The listing builds one solid part. Answer for the finished solid, in the listing's coordinates (mm). A direction names the side the tool comes from. Give positions to 0.01 mm unless a question says otherwise; leave off trailing zeros. Write each loop counter-clockwise with the first axis right and the second up, starting at its lowest first coordinate (ties: lowest second). Pieces come first, ordered by that corner, then holes. Notation, with made-up numbers: M 34.5,52 L 48.5,52 A21 ccw 48.5,63 Z; hole C 19.5,36 d10. An arc over 180 degrees is marked long. Return JSON: item names as keys, results as strings.
from build123d import *

# Parameters (mm, degrees)
SKETCH1_W             = 35.56
SKETCH1_H             = 35.56
BOSS_EXTRUDE1_DEPTH   = 6.35
CUT_EXTRUDE1_DEPTH    = 2.921
LPATTERN11_COUNT      = 2
LPATTERN11_PITCH      = 35.56
LPATTERN11_COUNT_DIR2 = 2
LPATTERN11_PITCH_DIR2 = 35.56
LPATTERN15_COUNT      = 2
LPATTERN15_PITCH      = 35.56
LPATTERN16_COUNT      = 2
LPATTERN16_PITCH      = 35.56
SKETCH20_W            = 3.175
SKETCH20_H            = 12.7
BOSS_EXTRUDE2_DEPTH   = 6.35
CUT_EXTRUDE2_DEPTH    = 76.700949135
SKETCH22_W            = 12.7
SKETCH22_H            = 3.175
BOSS_EXTRUDE3_DEPTH   = 6.35
CUT_EXTRUDE3_DEPTH    = 78.97065682
CUT_EXTRUDE4_DEPTH    = 78.97065682
CUT_EXTRUDE5_DEPTH    = 78.97065682


with BuildPart() as part:
    # Sketch1 → Boss-Extrude1 (new body)
    with BuildSketch(Plane(origin=(0, 0, 0), x_dir=(1, 0, 0), z_dir=(0, 1, 0))):
        Rectangle(SKETCH1_W, SKETCH1_H)
    boss_extrude1 = extrude(amount=BOSS_EXTRUDE1_DEPTH)

    # Sketch2 → Cut-Extrude1 (cut)
    with BuildSketch(Plane(origin=(0, 6.35, 0), x_dir=(1, 0, 0), z_dir=(0, 1, 0))):
        Polygon((0, 6.599113577), (-5.715, 3.299556788), (-5.715, -3.299556788), (0, -6.599113577), (5.715, -3.299556788), (5.715, 3.299556788), align=None)
    cut_extrude1 = extrude(amount=-CUT_EXTRUDE1_DEPTH, mode=Mode.SUBTRACT)

    # Sketch3 → 1/4 Clearance Hole1 (revolve, cut)
    with BuildSketch(Plane(origin=(0, 3.429, 0), x_dir=(0, 0, 1), z_dir=(1, 0, 0))):
        Polygon((0, 0), (0, 11.035817477), (3.57124, 8.89), (3.57124, 0), align=None)
    f_1_4_clearance_hole1 = revolve(axis=Axis((0, 9.779, 0), (0, -1, 0)), mode=Mode.SUBTRACT)

    # LPattern11: Boss-Extrude1, Cut-Extrude1, 1_4 Clearance Hole1 2 × 2
    with Locations(*[(-j * LPATTERN11_PITCH_DIR2, 0, i * LPATTERN11_PITCH) for i in range(LPATTERN11_COUNT) for j in range(LPATTERN11_COUNT_DIR2) if (i, j) != (0, 0)]):
        add(boss_extrude1)
        add(cut_extrude1, mode=Mode.SUBTRACT)
        add(f_1_4_clearance_hole1, mode=Mode.SUBTRACT)

    # Sketch15 → CBORE for #4 Socket Head Cap Screw5 (revolve, cut)
    with BuildSketch(Plane(origin=(0, 0, -11.557), x_dir=(0, 0, -1), z_dir=(1, 0, 0))):
        Polygon((0, 0), (0, 9.775187864), (1.4732, 8.89), (1.4732, 3.81), (2.794, 3.81), (2.794, 0), align=None)
    cbore_for_4_socket_head_cap_screw5 = revolve(axis=Axis((0, -6.35, -11.557), (0, 1, 0)), mode=Mode.SUBTRACT)

    # LPattern15: CBORE for #4 Socket Head Cap Screw5 ×2
    with Locations(*[(-i * LPATTERN15_PITCH, 0, 0) for i in range(1, LPATTERN15_COUNT)]):
        add(cbore_for_4_socket_head_cap_screw5, mode=Mode.SUBTRACT)

    # Sketch17 → CBORE for #4 Socket Head Cap Screw6 (revolve, cut)
    with BuildSketch(Plane(origin=(0, 0, 17.78), x_dir=(0, 0, -1), z_dir=(1, 0, 0))):
        Polygon((0, 0), (0, 9.775187864), (1.4732, 8.89), (1.4732, 3.81), (2.794, 3.81), (2.794, 0), align=None)
    cbore_for_4_socket_head_cap_screw6 = revolve(axis=Axis((0, -6.35, 17.78), (0, 1, 0)), mode=Mode.SUBTRACT)

    # LPattern16: CBORE for #4 Socket Head Cap Screw6 ×2
    with Locations(*[(-i * LPATTERN16_PITCH, 0, 0) for i in range(1, LPATTERN16_COUNT)]):
        add(cbore_for_4_socket_head_cap_screw6, mode=Mode.SUBTRACT)

    # Mirror1: CBORE for #4 Socket Head Cap Screw5 across plane
    add(cbore_for_4_socket_head_cap_screw5.mirror(Plane.XY.offset(17.78)), mode=Mode.SUBTRACT)

    # Mirror1 copy 1 sketch → Mirror1 copy 1 (revolve, cut)
    with BuildSketch(Plane(origin=(-35.56, 0, 47.117), x_dir=(0, 0, 1), z_dir=(1, 0, 0))):
        Polygon((0, 0), (0, -9.775187864), (1.4732, -8.89), (1.4732, -3.81), (2.794, -3.81), (2.794, 0), align=None)
    revolve(axis=Axis((-35.56, -6.35, 47.117), (0, -1, 0)), mode=Mode.SUBTRACT)

    # Sketch20 → Boss-Extrude2 (add)
    with BuildSketch(Plane(origin=(0, 0, 0), x_dir=(1, 0, 0), z_dir=(0, 1, 0))):
        with Locations((19.3675, 0)):
            Rectangle(SKETCH20_W, SKETCH20_H)
        with Locations((19.3675, -35.56)):
            Rectangle(SKETCH20_W, SKETCH20_H)
    extrude(amount=BOSS_EXTRUDE2_DEPTH)

    # Sketch21 → Cut-Extrude2 (cut, through all)
    with BuildSketch(Plane(origin=(0, 6.35, 0), x_dir=(1, 0, 0), z_dir=(0, 1, 0))):
        Polygon((20.955, -6.35), (17.78, -6.35), (17.78, -3.302), align=None)
        Polygon((20.955, 6.35), (17.78, 6.35), (17.78, 3.302), align=None)
        Polygon((20.955, -29.21), (17.78, -29.21), (17.78, -32.258), align=None)
        Polygon((20.955, -41.91), (17.78, -41.91), (17.78, -38.862), align=None)
    extrude(amount=-CUT_EXTRUDE2_DEPTH, mode=Mode.SUBTRACT)

    # Sketch22 → Boss-Extrude3 (add)
    with BuildSketch(Plane(origin=(0, 0, 0), x_dir=(1, 0, 0), z_dir=(0, 1, 0))):
        with Locations((-35.56, -54.9275)):
            Rectangle(SKETCH22_W, SKETCH22_H)
        with Locations((0, -54.9275)):
            Rectangle(SKETCH22_W, SKETCH22_H)
    extrude(amount=BOSS_EXTRUDE3_DEPTH)

    # Sketch23 → Cut-Extrude3 (cut, through all)
    with BuildSketch(Plane(origin=(0, 6.35, 0), x_dir=(1, 0, 0), z_dir=(0, 1, 0))):
        Polygon((-41.91, -56.515), (-41.91, -53.34), (-38.862, -53.34), align=None)
        Polygon((-29.21, -56.515), (-29.21, -53.34), (-32.258, -53.34), align=None)
        Polygon((-6.35, -56.515), (-6.35, -53.34), (-3.302, -53.34), align=None)
        Polygon((6.35, -56.515), (6.35, -53.34), (3.302, -53.34), align=None)
    extrude(amount=-CUT_EXTRUDE3_DEPTH, mode=Mode.SUBTRACT)

    # Sketch24 → Cut-Extrude4 (cut, through all)
    with BuildSketch(Plane(origin=(0, 6.35, 0), x_dir=(1, 0, 0), z_dir=(0, 1, 0))):
        Polygon((-53.34, 3.3655), (-53.34, -3.3655), (-50.165, -6.5913), (-50.165, 6.3627), align=None)
    cut_extrude4 = extrude(amount=-CUT_EXTRUDE4_DEPTH, mode=Mode.SUBTRACT)

    # Mirror2: Cut-Extrude4 across plane
    add(cut_extrude4.mirror(Plane.XY.offset(17.78)), mode=Mode.SUBTRACT)

    # Sketch25 → Cut-Extrude5 (cut, through all)
    with BuildSketch(Plane(origin=(0, 6.35, 0), x_dir=(1, 0, 0), z_dir=(0, 1, 0))):
        Polygon((-38.1, 17.78), (-33.02, 17.78), (-29.083, 14.605), (-42.037, 14.605), align=None)
        Polygon((-2.54, 17.78), (2.54, 17.78), (6.477, 14.605), (-6.477, 14.605), align=None)
    extrude(amount=-CUT_EXTRUDE5_DEPTH, mode=Mode.SUBTRACT)


solid = part.part
Item 1: Given pin 1 Ø6.5 at (x, z) = (-35.56, 35.56) entering from +Y; pin 2 Ø0.9 at (y, z) = (4.5, 35) entering from -X (3 decimals); pin 3 Ø3 at (x, y) = (10, 1.5) entering from +Z; pin 4 Ø2 at (y, z) = (5, 26) entering from +X, each flat-ended and moving along its own axis, determine where each tip first touches the part or whether it passes through.
Geometry results:
{"pin 1": "passes through", "pin 2": "stops at x = -50.165", "pin 3": "stops at z = 53.34", "pin 4": "stops at x = 17.78"}
Item 2: Determine the mould class of faces 4 (the flat face through (1, 3.81, -10)), 5 (the flat face through (-17, 0, 19)) for opening direction X: +X half, -X half, draft (parallel to the pull), parting line (faces both ways), or undercut.
Geometry results:
{"face 4": "undercut", "face 5": "draft"}
Item 3: A cutting plane is placed at A-A, the plane z = 17.78. Write down the section's boundary in (x, y).
Geometry results:
{"outline": "M -53.34,0 L -38.35,0 L -38.35,3.81 L -37.03,3.81 L -37.03,6.35 L -53.34,6.35 Z; M -34.09,3.81 L -32.77,3.81 L -32.77,0 L -2.79,0 L -2.79,3.81 L -1.47,3.81 L -1.47,6.35 L -34.09,6.35 Z; M 1.47,3.81 L 2.79,3.81 L 2.79,0 L 17.78,0 L 17.78,6.35 L 1.47,6.35 Z"}
Item 4: A cutting plane is placed at D-D, the plane z = 0. Write down the section's boundary in (x, y) (3 decimals).
Geometry results:
{"outline": "M -50.165,0 L -39.131,0 L -39.131,3.429 L -41.275,3.429 L -41.275,6.35 L -50.165,6.35 Z; M -31.989,0 L -3.571,0 L -3.571,3.429 L -5.715,3.429 L -5.715,6.35 L -29.845,6.35 L -29.845,3.429 L -31.989,3.429 Z; M 3.571,0 L 20.955,0 L 20.955,6.35 L 5.715,6.35 L 5.715,3.429 L 3.571,3.429 Z"}
Item 5: Find the intervals of material crossed by line 1 (Z direction, x = 0, y = 0.7) (3 decimals); line 2 (X direction, y = 4, z = 37) (3 decimals); line 3 (Z direction, x = -35.56, y = 5) (3 decimals), in increasing order.
Geometry results:
{"line 1": "z = -14.605 to -14.351, -8.763 to -3.571, 3.571 to 14.986, 20.574 to 31.989, 39.131 to 44.323, 49.911 to 56.515", "line 2": "x = -50.165 to -41.275, -29.845 to -5.715, 5.715 to 20.955", "line 3": "z = -14.605 to -13.03, -10.084 to -6.599, 6.599 to 16.307, 19.253 to 28.961, 42.159 to 45.644, 48.59 to 56.515"}
Item 6: A cutting plane is placed at C-C, the plane x = -28. Write down the section's boundary in (y, z).
Geometry results:
{"outline": "M 0,-17.78 L 6.35,-17.78 L 6.35,53.34 L 0,53.34 Z"}
Item 7: A cutting plane is placed at B-B, the plane y = 1. Count the separate pieces of the cut face and the enclosed holes in it, plus the area to 3 significant figures.
Geometry results:
{"separate pieces": "1", "enclosed holes": "10", "area": "4,750 mm2"}
Item 8: Which of the six approach directions +Z, -Z, +X, -X, +Y, -Y give full straight-line access (tool end or side, diameter ignored) to faces 1 (the flat face through (10, 3, 53.34)), 2 (the flat face through (-38.38, 4.91, -4.97)), 3 (the cylindrical face through (-35.683, 1.878, 44.326))?
Geometry results:
{"face 1": "+X, +Y, -Y", "face 2": "+Y", "face 3": "-Y"}
